```python
from build123d import *

# Parameters (mm, degrees)
F2_R = 1.5875
F3_R = 3.175


with BuildPart() as f1:
    # F0 (on Front) → F1 (revolve)
    with BuildSketch(Plane.XZ):
        with BuildLine():
            Line((3.175, 6.35), (3.175, 0))
            Line((3.175, 0), (20.6375, 0))
            Line((20.6375, 0), (20.6375, 4.7625))
            ThreePointArc((20.6375, 4.7625), (18.212016, 11.1125), (20.6375, 17.4625))
            Line((20.6375, 17.4625), (20.6375, 41.275))
            Line((20.6375, 41.275), (15.755542, 41.275))
            Line((15.755542, 41.275), (12.7, 6.35))
            Line((12.7, 6.35), (3.175, 6.35))
        make_face()
    revolve(axis=Axis((0, 0, 42.399504), (0, 0, 1)))

    # F2
    f2_edges = [f1.edges().sort_by_distance(p)[0] for p in [
        (-12.7, 0, 6.35),
    ]]
    fillet(f2_edges, radius=F2_R)

    # F3
    f3_edges = [f1.edges().sort_by_distance(p)[0] for p in [
        (-20.6375, 0, 17.4625),
        (-20.6375, 0, 4.7625),
    ]]
    fillet(f3_edges, radius=F3_R)


solid = f1.part
```
The listing builds one solid part. Answer for the finished solid, in the listing's coordinates (mm). A direction names the side the tool comes from. Round coordinates to 2 decimals unless told otherwise and drop trailing zeros. Order: outer loops, then holes, each group sorted by start corner. A loop starts at its lowest first (then second) coordinate and runs counter-clockwise, first axis right, second up. Notation, with made-up numbers: (45, 78) -> (93, 78) arc R9 cw to (93, 84) -> close; hole circle Ø6 at (87, 64.25). An arc over 180 degrees is marked (long way). Answer as CSV lines item,"result".
Q1. Which of the six approach directions +Z, -Z, +X, -X, +Y, -Y give full straight-line access (tool end or side, diameter ignored) to faces 4 (the flat face through (2, 3, 6.35)), 5 (the cylindrical face through (-4.474, -20.147, 30.085))?
Computed values:
face 4,"+Z"
face 5,"+Z, -Z"
Q2. A cutting plane is placed at A-A on z = 35.5. Determine the outline of the cut face in (x, y) (1 decimal).
Computed values:
outline,"circle Ø41.3 at (0, 0); hole circle Ø30.5 at (0, 0)"
Q3. For a pull along Y with two mould halves and no side action, classify faces 1 (the flat face through (-4.7, -15.2, 41.275)), 2 (the cylindrical face through (-4.474, -20.147, 1.849)), 3 (the conical face through (-1.86, 14.15, 24.3)) as +Y half, -Y half, draft (parallel to the pull), parting line (faces both ways), or undercut.
Computed values:
face 1,"draft"
face 2,"parting line"
face 3,"undercut"
Q4. Given pin 1 (1 mm diameter, centred on x = -3, z = 27.5, fed in from +Y); pin 2 (12 mm diameter, centred on x = 12, z = 22, fed in from -Y); pin 3 (4 mm diameter, centred on x = 0, y = 0, fed in from +Z); pin 4 (6 mm diameter, centred on y = 3, z = 9, fed in from -X), each flat-ended and moving along its own axis, determine where each tip first touches the part or whether it passes through.
Computed values:
pin 1,"stops at y = 20.49"
pin 2,"stops at y = -19.75"
pin 3,"passes through"
pin 4,"stops at x = -19.52"
Q5. Consider line 1 (Y direction, x = 0, z = 3) (1 decimal); line 2 (X direction, y = -7.5, z = 30); line 3 (Z direction, x = -5, y = -1.5). Determine where each line is inside the solid, lowest interval first. Write a range as from..to.
Computed values:
line 1,"y = -20.6..-3.2, 3.2..20.6"
line 2,"x = -19.23..-12.72, 12.72..19.23"
line 3,"z = 0..6.35"
Q6. A cutting plane is placed at B-B on z = 12.5. Determine the outline of the cut face in (x, y), plus the area to 3 significant figures.
Computed values:
outline,"circle Ø36.63 at (0, 0); hole circle Ø26.48 at (0, 0)"
area,"503 mm^2"
